Geometry: final body of the model. Coordinates: model frame, mm. Face numbers are marked on the shaded views. A direction names the side the tool comes from. Give positions to 0.01 mm unless a question says otherwise; leave off trailing zeros. Order: outer loops, then holes, each group sorted by start corner. A loop starts at its lowest first (then second) coordinate and runs counter-clockwise, first axis right, second up. Notation, with made-up numbers: (43.25, -9.75) -> (62.25, -9.75) arc R17 ccw to (62.25, 13.25) -> close; hole circle Ø1 at (29, 47). An arc over 180 degrees is marked (long way). One line per question, with ' | ' between items. Start each with the question number.
(1) First-contact query: pin 1 Ø0.8 at (y, z) = (7.5, 14.5) entering from -X; pin 2 Ø2 at (y, z) = (3, 3) entering from -X; pin 3 Ø1.2 at (y, z) = (-7.5, 12.5) entering from -X. Flat tips, straight axial feed; report the tip coordinate or a pass-through.
(2) Section B-B (z = 16.5). Return loops of the section in (x, y).
(3) Ray query, L1, parallel to Z at x = -7.5, y = 10; L2, parallel to Y at x = 0, z = 7.25; L3, parallel to Y at x = 0, z = 22.45. Return the intervals inside material, ascending.
(4) Section D-D (x = 16). Return loops of the section in (y, z).
(5) Set-up query: the marked faces 1 and 2. Return all of +Z, -Z, +X, -X, +Y, -Y with unobstructed straight access to the full face (end or side cutting, diameter ignored); none if empty.
(6) Section C-C (x = 0). Return loops of the section in (y, z), then the cut area to 3 significant figures.
(7) Mould query, pull axis Y, two halves, no side actions, for the marked faces 3, 4 and 5. Classes: +Y half, -Y half, draft (parallel to the pull), parting line (faces both ways), or undercut.
(8) Section A-A (y = 0). Return loops of the section in (x, z), then the cut area to 3 significant figures.
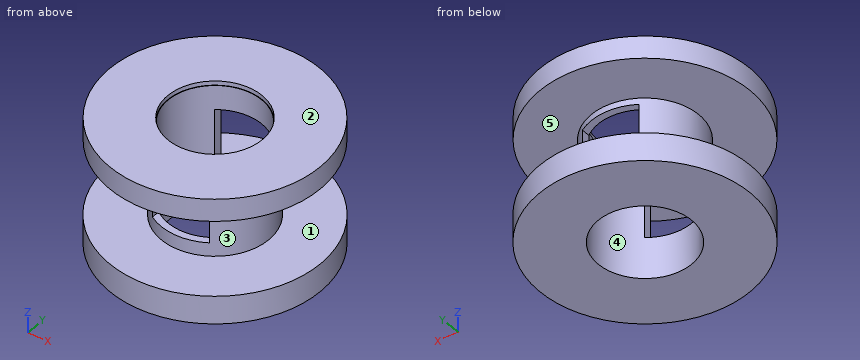
```python
from build123d import *

# Parameters (mm, degrees)
F0_R          = 19.05
F0_R_2        = 9.7365901145
F1_DEPTH      = 5.08
F0_R_3        = 8.4665901145
F2_DEPTH      = 22.098
F4_START      = 18.796
F3_R          = 19.0205211377
F3_R_2        = 8.5460755938
F4_DEPTH      = 4.064
F5_W          = 10.16
F5_H          = 10.16
F6_DEPTH      = 13.716
F6_DEPTH_BACK = 12.446


with BuildPart() as f1:
    # F0 (on Top) → F1 (new body)
    with BuildSketch(Plane.XY):
        Circle(F0_R)
        Circle(F0_R_2, mode=Mode.SUBTRACT)
    extrude(amount=F1_DEPTH)

    # F0 (on Top) → F2 (join)
    with BuildSketch(Plane.XY):
        Circle(F0_R_2)
        Circle(F0_R_3, mode=Mode.SUBTRACT)
    extrude(amount=F2_DEPTH)

    # F3 (on Top) → F4 (join)
    with BuildSketch(Plane.XY.offset(F4_START)):
        Circle(F3_R)
        Circle(F3_R_2, mode=Mode.SUBTRACT)
    extrude(amount=F4_DEPTH)

    # F5 (on Front) → F6 (cut, two sides)
    with BuildSketch(Plane.XZ) as f6_sk:
        with Locations((0.0056111868, 12.6004907916)):
            Rectangle(F5_W, F5_H)
    extrude(amount=-F6_DEPTH, mode=Mode.SUBTRACT)
    extrude(f6_sk.sketch, amount=F6_DEPTH_BACK, mode=Mode.SUBTRACT)


solid = f1.part
```
Response:
1) pin 1: stops at x = -6.66 | pin 2: stops at x = -18.94 | pin 3: stops at x = -6.87
2) outline: (-5.07, -8.31) -> (-5.07, -6.78) arc R8.47 cw to (-5.07, 6.78) -> (-5.07, 8.31) arc R9.74 ccw to start; (5.09, -8.3) arc R9.74 ccw to (5.09, 8.3) -> (5.09, 6.77) arc R8.47 cw to (5.09, -6.77) -> close
3) L1: z = 0 to 5.08, 18.8 to 22.86 | L2: y = -9.74 to -8.47, 8.47 to 9.74 | L3: y = -19.02 to -8.55, 8.55 to 19.02
4) outline: (-10.34, 0) -> (10.34, 0) -> (10.34, 5.08) -> (-10.34, 5.08) -> close; (-10.28, 18.8) -> (10.28, 18.8) -> (10.28, 22.86) -> (-10.28, 22.86) -> close
5) face 1: none | face 2: +Z, +X, -X, +Y, -Y
6) outline: (-19.05, 0) -> (-8.47, 0) -> (-8.47, 7.52) -> (-9.74, 7.52) -> (-9.74, 5.08) -> (-19.05, 5.08) -> close; (-19.02, 18.8) -> (-9.74, 18.8) -> (-9.74, 17.68) -> (-8.47, 17.68) -> (-8.47, 22.1) -> (-8.55, 22.1) -> (-8.55, 22.86) -> (-19.02, 22.86) -> close; (8.47, 0) -> (19.05, 0) -> (19.05, 5.08) -> (9.74, 5.08) -> (9.74, 7.52) -> (8.47, 7.52) -> close; (8.47, 17.68) -> (9.74, 17.68) -> (9.74, 18.8) -> (19.02, 18.8) -> (19.02, 22.86) -> (8.55, 22.86) -> (8.55, 22.1) -> (8.47, 22.1) -> close | area: 202 mm^2
7) face 3: parting line | face 4: undercut | face 5: draft
8) outline: (-19.05, 0) -> (-8.47, 0) -> (-8.47, 22.1) -> (-8.55, 22.1) -> (-8.55, 22.86) -> (-19.02, 22.86) -> (-19.02, 18.8) -> (-9.74, 18.8) -> (-9.74, 5.08) -> (-19.05, 5.08) -> close; (8.47, 0) -> (19.05, 0) -> (19.05, 5.08) -> (9.74, 5.08) -> (9.74, 18.8) -> (19.02, 18.8) -> (19.02, 22.86) -> (8.55, 22.86) -> (8.55, 22.1) -> (8.47, 22.1) -> close | area: 228 mm^2
